from build123d import *

# Parameters (mm, degrees)
BOSS_EXTRUDE2_DEPTH   = 3.24
BOSS_EXTRUDE2_2_DEPTH = 3.24
SKETCH1_5_W           = 37.369599927
SKETCH1_5_H           = 20
BOSS_EXTRUDE3_DEPTH   = 11.78
SKETCH2_R             = 4.04
BOSS_EXTRUDE4_DEPTH   = 4.9
FILLET5_R             = 2.5
SKETCH1_6_W           = 37.369599927
SKETCH1_6_H           = 20
BOSS_EXTRUDE8_DEPTH   = 16.74
BOSS_EXTRUDE9_DEPTH   = 5
SKETCH7_W             = 37.369599927
SKETCH7_H             = 20
BOSS_EXTRUDE10_DEPTH  = 9.5
FILLET6_R             = 0.5
CUT_EXTRUDE2_DEPTH    = 1.66


with BuildPart() as part:
    # Sketch1 → Boss-Extrude2 (new body)
    with BuildSketch(Plane(origin=(0, 0, 0), x_dir=(1, 0, 0), z_dir=(0, 1, 0))):
        with BuildLine():
            Line((-18.219599927, -10), (-18.219599927, 10))
            Line((-18.219599927, 10), (-23.852132603, 10))
            ThreePointArc((-23.852132603, 10), (-25.619899556, 9.267766953), (-26.352132603, 7.5))
            Line((-26.352132603, 7.5), (-26.352132603, 5.968724559))
            ThreePointArc((-26.352132603, 5.968724559), (-22.261829683, 5.035135291), (-26.319599927, 3.96898917))
            Line((-26.319599927, 3.96898917), (-26.319599927, -4))
            ThreePointArc((-26.319599927, -4), (-22.245024256, -5), (-26.319599927, -6))
            Line((-26.319599927, -6), (-26.319599927, -7.5))
            ThreePointArc((-26.319599927, -7.5), (-25.58736688, -9.267766953), (-23.819599927, -10))
            Line((-23.819599927, -10), (-18.219599927, -10))
        make_face()
    extrude(amount=BOSS_EXTRUDE2_DEPTH)



with BuildPart() as body_2:
    # Sketch1 → Boss-Extrude2 2 (new body)
    with BuildSketch(Plane(origin=(0, 0, 0), x_dir=(1, 0, 0), z_dir=(0, 1, 0))):
        with BuildLine():
            ThreePointArc((27.25, 4), (23.175424329, 5), (27.25, 6))
            Line((27.25, 6), (27.25, 7.5))
            ThreePointArc((27.25, 7.5), (26.517766953, 9.267766953), (24.75, 10))
            Line((24.75, 10), (19.15, 10))
            Line((19.15, 10), (19.15, -10))
            Line((19.15, -10), (24.75, -10))
            ThreePointArc((24.75, -10), (26.517766953, -9.267766953), (27.25, -7.5))
            Line((27.25, -7.5), (27.25, -6))
            ThreePointArc((27.25, -6), (23.175424329, -5), (27.25, -4))
            Line((27.25, -4), (27.25, 4))
        make_face()
    extrude(amount=BOSS_EXTRUDE2_2_DEPTH)


with BuildPart() as part_1:
    add(part.part)

    add(body_2.part)  # Boss-Extrude3 merges body 2
    # Sketch1_5 → Boss-Extrude3 (add)
    with BuildSketch(Plane(origin=(0, 0, 0), x_dir=(1, 0, 0), z_dir=(0, 1, 0))):
        with Locations((0.465200037, 0)):
            Rectangle(SKETCH1_5_W, SKETCH1_5_H)
    extrude(amount=BOSS_EXTRUDE3_DEPTH)

    # Sketch2 → Boss-Extrude4 (add)
    with BuildSketch(Plane(origin=(0, 11.78, 0), x_dir=(1, 0, 0), z_dir=(0, 1, 0))):
        with Locations(Location((9.316469078, 0, 0), (0, 0, 270))):
            Circle(SKETCH2_R)
    extrude(amount=BOSS_EXTRUDE4_DEPTH)

    # Fillet5
    fillet5_edges = [part_1.edges().sort_by_distance(p)[0] for p in [
        (19.15, 11.78, 0),
        (0.465200037, 11.78, -10),
        (-18.219599927, 11.78, 0),
        (0.465200037, 11.78, 10),
        (9.316469078, 11.78, -4.04),
    ]]
    fillet(fillet5_edges, radius=FILLET5_R)

    # Sketch1_6 → Boss-Extrude8 (add)
    with BuildSketch(Plane(origin=(0, 0, 0), x_dir=(1, 0, 0), z_dir=(0, 1, 0))):
        with Locations((0.465200037, 0)):
            Rectangle(SKETCH1_6_W, SKETCH1_6_H)
    extrude(amount=-BOSS_EXTRUDE8_DEPTH)

    # Sketch6 → Boss-Extrude9 (add)
    with BuildSketch(Plane(origin=(19.15, 0, 0), x_dir=(0, 0, -1), z_dir=(1, 0, 0))):
        Polygon((-2.757398298, -15.385544214), (4.924102175, -16.74), (4.229509465, -20.679231012), (-3.451991009, -19.324775226), align=None)
    extrude(amount=BOSS_EXTRUDE9_DEPTH)

    # Sketch7 → Boss-Extrude10 (add)
    with BuildSketch(Plane.XZ.offset(16.74)):
        with Locations((0.465200037, 0)):
            Rectangle(SKETCH7_W, SKETCH7_H)
    extrude(amount=BOSS_EXTRUDE10_DEPTH)

    # Fillet6
    fillet6_edges = [part_1.edges().sort_by_distance(p)[0] for p in [
        (-18.219599927, -26.24, 0),
        (0.465200037, -26.24, -10),
        (19.15, -26.24, 0),
        (0.465200037, -26.24, 10),
    ]]
    fillet(fillet6_edges, radius=FILLET6_R)

    # Sketch8 → Cut-Extrude2 (cut)
    with BuildSketch(Plane.XZ.offset(26.24)):
        with BuildLine():
            Line((16.22, 5.04), (18.65, 5.04))
            Line((18.65, 5.04), (18.65, 9.5))
            Line((18.65, 9.5), (14.19, 9.5))
            Line((14.19, 9.5), (14.19, 7.07))
            ThreePointArc((14.19, 7.07), (14.784573234, 5.634573234), (16.22, 5.04))
        make_face()
        with BuildLine():
            Line((-13.259599927, 7.07), (-13.259599927, 9.5))
            Line((-13.259599927, 9.5), (-17.719599927, 9.5))
            Line((-17.719599927, 9.5), (-17.719599927, 5.04))
            Line((-17.719599927, 5.04), (-15.289599927, 5.04))
            ThreePointArc((-15.289599927, 5.04), (-13.854173161, 5.634573234), (-13.259599927, 7.07))
        make_face()
        with BuildLine():
            Line((18.65, -9.5), (18.65, -5.04))
            Line((18.65, -5.04), (16.22, -5.04))
            ThreePointArc((16.22, -5.04), (14.784573234, -5.634573234), (14.19, -7.07))
            Line((14.19, -7.07), (14.19, -9.5))
            Line((14.19, -9.5), (18.65, -9.5))
        make_face()
        with BuildLine():
            Line((-15.289599927, -5.04), (-17.719599927, -5.04))
            Line((-17.719599927, -5.04), (-17.719599927, -9.5))
            Line((-17.719599927, -9.5), (-13.259599927, -9.5))
            Line((-13.259599927, -9.5), (-13.259599927, -7.07))
            ThreePointArc((-13.259599927, -7.07), (-13.854173161, -5.634573234), (-15.289599927, -5.04))
        make_face()
    extrude(amount=-CUT_EXTRUDE2_DEPTH, mode=Mode.SUBTRACT)


solid = part_1.part
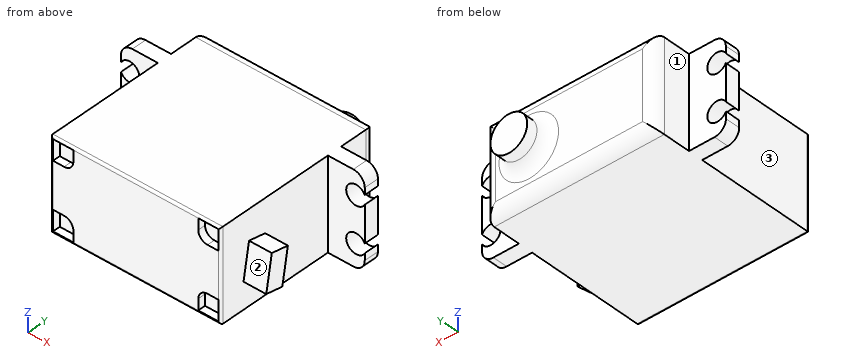
Geometry check sheet. Reference: the model listing, model coordinates, mm. Face numbers are marked on the shaded views. A direction names the side the tool comes from. Give positions to 0.01 mm unless a question says otherwise; leave off trailing zeros. Loops run counter-clockwise (first coordinate to the right, second up) from the corner with the lowest first, then second, coordinate; pieces in that order, holes last.
(1) Depth check by flat-ended pin: pin 1 Ø4 at (y, z) = (-19, 0) entering from +X; pin 2 Ø1.3 at (y, z) = (-25.5, -8) entering from -X; pin 3 Ø3 at (x, z) = (6, -7.5) entering from +Y; pin 4 Ø5 at (x, z) = (17, -8.5) entering from -Y. Enter the tip coordinate at first touch or a pass-through.
From the geometry:
pin 1: stops at x = 24.15
pin 2: stops at x = -18.22
pin 3: stops at y = 11.78
pin 4: stops at y = -26.24
(2) Section check C-C on z = 0. Record the cut outline in (x, y).
From the geometry:
outline: (-26.32, 0) - (-18.22, 0) - (-18.22, -25.74) arc R0.5 ccw to (-17.72, -26.24) - (18.65, -26.24) arc R0.5 ccw to (19.15, -25.74) - (19.15, -19.93) - (24.15, -19.93) - (24.15, -15.87) - (19.15, -15.87) - (19.15, 0) - (27.25, 0) - (27.25, 3.24) - (19.15, 3.24) - (19.15, 9.28) arc R2.5 ccw to (16.65, 11.78) - (15.86, 11.78) arc R2.5 cw to (13.36, 14.28) - (13.36, 16.68) - (5.28, 16.68) - (5.28, 14.28) arc R2.5 cw to (2.78, 11.78) - (-15.72, 11.78) arc R2.5 ccw to (-18.22, 9.28) - (-18.22, 3.24) - (-26.32, 3.24) - close
(3) Thickness scan on L1, parallel to X at y = -15, z = -8; L2, parallel to X at y = 2, z = -5; L3, parallel to Y at x = 24, z = 7.5. Record the ranges inside material, lowest first.
From the geometry:
L1: x = -18.22 to 19.15
L2: x = -22.26 to 23.18
L3: y = 0 to 3.24
(4) Section check B-B on x = 0. Record the cut outline in (y, z).
From the geometry:
outline: (-26.24, -9.5) arc R0.5 ccw to (-25.74, -10) - (9.28, -10) arc R2.5 ccw to (11.78, -7.5) - (11.78, 7.5) arc R2.5 ccw to (9.28, 10) - (-25.74, 10) arc R0.5 ccw to (-26.24, 9.5) - close
(5) Set-up check for the marked faces 1, 2 and 3: record each of +Z, -Z, +X, -X, +Y, -Y from which the full face is reachable in a straight line by a thin tool's end or side.
From the geometry:
face 1: +Z, -Z, -X, +Y
face 2: +Z, +X, -Y
face 3: +Z, -Z, -X, -Y
(6) Section check D-D on x = -21. Record the cut outline in (y, z).
From the geometry:
outline: (0, -10) - (3.24, -10) - (3.24, 10) - (0, 10) - close
(7) Section check A-A on y = 2.5. Record the cut outline in (x, z).
From the geometry:
outline: (-26.35, -7.5) arc R2.5 ccw to (-23.85, -10) - (24.75, -10) arc R2.5 ccw to (27.25, -7.5) - (27.25, -6) arc R2.16 cw (long way) to (27.25, -4) - (27.25, 4) arc R2.16 cw (long way) to (27.25, 6) - (27.25, 7.5) arc R2.5 ccw to (24.75, 10) - (-23.82, 10) arc R2.5 ccw to (-26.32, 7.5) - (-26.32, 6) arc R2.16 cw (long way) to (-26.32, 4) - (-26.32, -3.97) arc R2.16 cw (long way) to (-26.35, -5.97) - close
